from build123d import *

# Parameters (mm, degrees)
F1_DEPTH = 25.4


with BuildPart() as f1:
    # F0 (on Front) → F1 (new body)
    with BuildSketch(Plane.XZ):
        with BuildLine():
            Line((-18.234044, -41.093612), (-33.907204, -68.240322))
            ThreePointArc((-33.907204, -68.240322), (-17.414469, -74.183396), (0, -76.2))
            Line((0, -76.2), (0, -44.45))
            ThreePointArc((0, -44.45), (-9.187875, -43.490061), (-17.97891, -40.651707))
            ThreePointArc((-17.97891, -40.651707), (-18.100554, -40.876079), (-18.234044, -41.093612))
        make_face()
        with BuildLine():
            Line((0, -44.45), (0, -76.2))
            ThreePointArc((0, -76.2), (17.414469, -74.183396), (33.907204, -68.240322))
            Line((33.907204, -68.240322), (18.234044, -41.093612))
            ThreePointArc((18.234044, -41.093612), (18.100554, -40.876079), (17.97891, -40.651707))
            ThreePointArc((17.97891, -40.651707), (9.187875, -43.490061), (0, -44.45))
        make_face()
        with BuildLine():
            Line((-17.97891, -40.651707), (-18.234044, -41.093612))
            ThreePointArc((-18.234044, -41.093612), (-18.100554, -40.876079), (-17.97891, -40.651707))
        make_face()
        with BuildLine():
            Line((0, -20.6375), (0, -44.45))
            ThreePointArc((0, -44.45), (9.187875, -43.490061), (17.97891, -40.651707))
            ThreePointArc((17.97891, -40.651707), (17.659459, -37.139382), (19.84375, -34.370383))
            Line((19.84375, -34.370383), (10.31875, -17.872599))
            ThreePointArc((10.31875, -17.872599), (5.341378, -19.934294), (0, -20.6375))
        make_face()
        with BuildLine():
            ThreePointArc((-17.97891, -40.651707), (-9.187875, -43.490061), (0, -44.45))
            Line((0, -44.45), (0, -20.6375))
            ThreePointArc((0, -20.6375), (-5.341378, -19.934294), (-10.31875, -17.872599))
            Line((-10.31875, -17.872599), (-19.84375, -34.370383))
            ThreePointArc((-19.84375, -34.370383), (-17.659459, -37.139382), (-17.97891, -40.651707))
        make_face()
        with BuildLine():
            ThreePointArc((17.97891, -40.651707), (18.100554, -40.876079), (18.234044, -41.093612))
            Line((18.234044, -41.093612), (17.97891, -40.651707))
        make_face()
        with BuildLine():
            ThreePointArc((-26.215956, -35.896046), (-23.333919, -33.863231), (-19.84375, -34.370383))
            Line((-19.84375, -34.370383), (-10.31875, -17.872599))
            ThreePointArc((-10.31875, -17.872599), (-14.592916, -14.592916), (-17.872599, -10.31875))
            Line((-17.872599, -10.31875), (-38.494829, -22.225))
            ThreePointArc((-38.494829, -22.225), (-33.06956, -29.701964), (-26.215956, -35.896046))
        make_face()
        with BuildLine():
            Line((10.31875, -17.872599), (19.84375, -34.370383))
            ThreePointArc((19.84375, -34.370383), (23.333919, -33.863231), (26.215956, -35.896046))
            ThreePointArc((26.215956, -35.896046), (33.06956, -29.701964), (38.494829, -22.225))
            Line((38.494829, -22.225), (17.872599, -10.31875))
            ThreePointArc((17.872599, -10.31875), (14.592916, -14.592916), (10.31875, -17.872599))
        make_face()
        with BuildLine():
            Line((-26.47109, -36.337951), (-26.215956, -35.896046))
            ThreePointArc((-26.215956, -35.896046), (-26.349446, -36.113579), (-26.47109, -36.337951))
        make_face()
        with BuildLine():
            ThreePointArc((-26.47109, -36.337951), (-26.349446, -36.113579), (-26.215956, -35.896046))
            ThreePointArc((-26.215956, -35.896046), (-33.06956, -29.701964), (-38.494829, -22.225))
            Line((-38.494829, -22.225), (-65.991136, -38.1))
            ThreePointArc((-65.991136, -38.1), (-55.537471, -52.173071), (-42.14425, -63.484661))
            Line((-42.14425, -63.484661), (-26.47109, -36.337951))
        make_face()
        with BuildLine():
            ThreePointArc((38.494829, -22.225), (33.06956, -29.701964), (26.215956, -35.896046))
            ThreePointArc((26.215956, -35.896046), (26.349446, -36.113579), (26.47109, -36.337951))
            Line((26.47109, -36.337951), (42.14425, -63.484661))
            ThreePointArc((42.14425, -63.484661), (55.537471, -52.173071), (65.991136, -38.1))
            Line((65.991136, -38.1), (38.494829, -22.225))
        make_face()
        with BuildLine():
            ThreePointArc((26.47109, -36.337951), (26.349446, -36.113579), (26.215956, -35.896046))
            Line((26.215956, -35.896046), (26.47109, -36.337951))
        make_face()
        with BuildLine():
            Line((-38.494829, -22.225), (-17.872599, -10.31875))
            ThreePointArc((-17.872599, -10.31875), (-19.934294, -5.341378), (-20.6375, 0))
            Line((-20.6375, 0), (-39.6875, 0))
            ThreePointArc((-39.6875, 0), (-40.993377, -3.276151), (-44.194866, -4.755661))
            ThreePointArc((-44.194866, -4.755661), (-42.257436, -13.788097), (-38.494829, -22.225))
        make_face()
        with BuildLine():
            ThreePointArc((20.6375, 0), (19.934294, -5.341378), (17.872599, -10.31875))
            Line((17.872599, -10.31875), (38.494829, -22.225))
            ThreePointArc((38.494829, -22.225), (42.257436, -13.788097), (44.194866, -4.755661))
            ThreePointArc((44.194866, -4.755661), (40.993377, -3.276151), (39.6875, 0))
            Line((39.6875, 0), (20.6375, 0))
        make_face()
        with BuildLine():
            Line((0, 44.45), (0, 20.6375))
            ThreePointArc((0, 20.6375), (5.341378, 19.934294), (10.31875, 17.872599))
            Line((10.31875, 17.872599), (19.84375, 34.370383))
            ThreePointArc((19.84375, 34.370383), (17.659459, 37.139382), (17.97891, 40.651707))
            ThreePointArc((17.97891, 40.651707), (9.187875, 43.490061), (0, 44.45))
        make_face()
        with BuildLine():
            ThreePointArc((-10.31875, 17.872599), (-5.341378, 19.934294), (0, 20.6375))
            Line((0, 20.6375), (0, 44.45))
            ThreePointArc((0, 44.45), (-9.187875, 43.490061), (-17.97891, 40.651707))
            ThreePointArc((-17.97891, 40.651707), (-17.659459, 37.139382), (-19.84375, 34.370383))
            Line((-19.84375, 34.370383), (-10.31875, 17.872599))
        make_face()
        with BuildLine():
            ThreePointArc((17.872599, 10.31875), (19.934294, 5.341378), (20.6375, 0))
            Line((20.6375, 0), (39.6875, 0))
            ThreePointArc((39.6875, 0), (40.993377, 3.276151), (44.194866, 4.755661))
            ThreePointArc((44.194866, 4.755661), (42.257436, 13.788097), (38.494829, 22.225))
            Line((38.494829, 22.225), (17.872599, 10.31875))
        make_face()
        with BuildLine():
            Line((-39.6875, 0), (-20.6375, 0))
            ThreePointArc((-20.6375, 0), (-19.934294, 5.341378), (-17.872599, 10.31875))
            Line((-17.872599, 10.31875), (-38.494829, 22.225))
            ThreePointArc((-38.494829, 22.225), (-42.257436, 13.788097), (-44.194866, 4.755661))
            ThreePointArc((-44.194866, 4.755661), (-40.993377, 3.276151), (-39.6875, 0))
        make_face()
        with BuildLine():
            ThreePointArc((-17.872599, 10.31875), (-14.592916, 14.592916), (-10.31875, 17.872599))
            Line((-10.31875, 17.872599), (-19.84375, 34.370383))
            ThreePointArc((-19.84375, 34.370383), (-23.333919, 33.863231), (-26.215956, 35.896046))
            ThreePointArc((-26.215956, 35.896046), (-33.06956, 29.701964), (-38.494829, 22.225))
            Line((-38.494829, 22.225), (-17.872599, 10.31875))
        make_face()
        with BuildLine():
            Line((19.84375, 34.370383), (10.31875, 17.872599))
            ThreePointArc((10.31875, 17.872599), (14.592916, 14.592916), (17.872599, 10.31875))
            Line((17.872599, 10.31875), (38.494829, 22.225))
            ThreePointArc((38.494829, 22.225), (33.06956, 29.701964), (26.215956, 35.896046))
            ThreePointArc((26.215956, 35.896046), (23.333919, 33.863231), (19.84375, 34.370383))
        make_face()
        with BuildLine():
            Line((-65.991136, -38.1), (-38.494829, -22.225))
            ThreePointArc((-38.494829, -22.225), (-42.257436, -13.788097), (-44.194866, -4.755661))
            ThreePointArc((-44.194866, -4.755661), (-44.45, -4.7625), (-44.705134, -4.755661))
            Line((-44.705134, -4.755661), (-76.051454, -4.755661))
            ThreePointArc((-76.051454, -4.755661), (-72.95194, -22.010325), (-65.991136, -38.1))
        make_face()
        with BuildLine():
            ThreePointArc((44.194866, -4.755661), (42.257436, -13.788097), (38.494829, -22.225))
            Line((38.494829, -22.225), (65.991136, -38.1))
            ThreePointArc((65.991136, -38.1), (72.95194, -22.010325), (76.051454, -4.755661))
            Line((76.051454, -4.755661), (44.705134, -4.755661))
            ThreePointArc((44.705134, -4.755661), (44.45, -4.7625), (44.194866, -4.755661))
        make_face()
        with BuildLine():
            ThreePointArc((-17.97891, 40.651707), (-9.187875, 43.490061), (0, 44.45))
            Line((0, 44.45), (0, 76.2))
            ThreePointArc((0, 76.2), (-17.414469, 74.183396), (-33.907204, 68.240322))
            Line((-33.907204, 68.240322), (-18.234044, 41.093612))
            ThreePointArc((-18.234044, 41.093612), (-18.100554, 40.876079), (-17.97891, 40.651707))
        make_face()
        with BuildLine():
            Line((0, 76.2), (0, 44.45))
            ThreePointArc((0, 44.45), (9.187875, 43.490061), (17.97891, 40.651707))
            ThreePointArc((17.97891, 40.651707), (18.100554, 40.876079), (18.234044, 41.093612))
            Line((18.234044, 41.093612), (33.907204, 68.240322))
            ThreePointArc((33.907204, 68.240322), (17.414469, 74.183396), (0, 76.2))
        make_face()
        with BuildLine():
            ThreePointArc((-44.194866, 4.755661), (-42.257436, 13.788097), (-38.494829, 22.225))
            Line((-38.494829, 22.225), (-65.991136, 38.1))
            ThreePointArc((-65.991136, 38.1), (-72.95194, 22.010325), (-76.051454, 4.755661))
            Line((-76.051454, 4.755661), (-44.705134, 4.755661))
            ThreePointArc((-44.705134, 4.755661), (-44.45, 4.7625), (-44.194866, 4.755661))
        make_face()
        with BuildLine():
            Line((-65.991136, 38.1), (-38.494829, 22.225))
            ThreePointArc((-38.494829, 22.225), (-33.06956, 29.701964), (-26.215956, 35.896046))
            ThreePointArc((-26.215956, 35.896046), (-26.349446, 36.113579), (-26.47109, 36.337951))
            Line((-26.47109, 36.337951), (-42.14425, 63.484661))
            ThreePointArc((-42.14425, 63.484661), (-55.537471, 52.173071), (-65.991136, 38.1))
        make_face()
        with BuildLine():
            ThreePointArc((26.215956, 35.896046), (33.06956, 29.701964), (38.494829, 22.225))
            Line((38.494829, 22.225), (65.991136, 38.1))
            ThreePointArc((65.991136, 38.1), (55.537471, 52.173071), (42.14425, 63.484661))
            Line((42.14425, 63.484661), (26.47109, 36.337951))
            ThreePointArc((26.47109, 36.337951), (26.349446, 36.113579), (26.215956, 35.896046))
        make_face()
        with BuildLine():
            Line((65.991136, 38.1), (38.494829, 22.225))
            ThreePointArc((38.494829, 22.225), (42.257436, 13.788097), (44.194866, 4.755661))
            ThreePointArc((44.194866, 4.755661), (44.45, 4.7625), (44.705134, 4.755661))
            Line((44.705134, 4.755661), (76.051454, 4.755661))
            ThreePointArc((76.051454, 4.755661), (72.95194, 22.010325), (65.991136, 38.1))
        make_face()
        with BuildLine():
            ThreePointArc((-44.705134, -4.755661), (-44.45, -4.7625), (-44.194866, -4.755661))
            Line((-44.194866, -4.755661), (-44.705134, -4.755661))
        make_face()
        with BuildLine():
            Line((44.705134, -4.755661), (44.194866, -4.755661))
            ThreePointArc((44.194866, -4.755661), (44.45, -4.7625), (44.705134, -4.755661))
        make_face()
        with BuildLine():
            ThreePointArc((18.234044, 41.093612), (18.100554, 40.876079), (17.97891, 40.651707))
            Line((17.97891, 40.651707), (18.234044, 41.093612))
        make_face()
        with BuildLine():
            Line((-18.234044, 41.093612), (-17.97891, 40.651707))
            ThreePointArc((-17.97891, 40.651707), (-18.100554, 40.876079), (-18.234044, 41.093612))
        make_face()
        with BuildLine():
            ThreePointArc((44.705134, 4.755661), (44.45, 4.7625), (44.194866, 4.755661))
            Line((44.194866, 4.755661), (44.705134, 4.755661))
        make_face()
        with BuildLine():
            Line((-44.705134, 4.755661), (-44.194866, 4.755661))
            ThreePointArc((-44.194866, 4.755661), (-44.45, 4.7625), (-44.705134, 4.755661))
        make_face()
        with BuildLine():
            ThreePointArc((-26.47109, 36.337951), (-26.349446, 36.113579), (-26.215956, 35.896046))
            Line((-26.215956, 35.896046), (-26.47109, 36.337951))
        make_face()
        with BuildLine():
            Line((26.47109, 36.337951), (26.215956, 35.896046))
            ThreePointArc((26.215956, 35.896046), (26.349446, 36.113579), (26.47109, 36.337951))
        make_face()
    extrude(amount=F1_DEPTH)


solid = f1.part
Could you check a few things on this model? Use its own coordinates, in mm. A direction names the side the tool comes from. Coordinates: 2 decimals unless noted, no trailing zeros. Write each loop counter-clockwise with the first axis right and the second up, starting at its lowest first coordinate (ties: lowest second). Pieces come first, ordered by that corner, then holes. Notation, with made-up numbers: (43, -3.75) - (69, -3.75) arc R23 cw to (69, 22.25) - close; hole circle Ø8 at (-37.75, 55). An arc over 180 degrees is marked (long way). Put each result on its own line as item: value. Start each with the question number.
Q1. I want a section at B-B on z = -53. Write out the boundary of the cut face in (x, y), plus the area to 3 significant figures.
Q2. I want a section at D-D on z = 60.5. Write out the boundary of the cut face in (x, y).
Q3. Please list where these lines run through material, in increasing order: L1, parallel to X at y = -17.5, z = 49; L2, parallel to X at y = -6.5, z = 46.5; L3, parallel to X at y = -14.25, z = 0.5.
Q4. I want a section at A-A on x = 47. Write out the boundary of the cut face in (y, z), plus the area to 3 significant figures.
Q5. Which directions (+Z, -Z, +X, -X, +Y, -Y) give clear straight access to the entire face, cutting with the end or side of a thin tool? Please do faces 1 (the flat face through (-60, -13, -4.756)), 2 (the flat face through (16, 0, -16)), 3 (the flat face through (60, -13, -4.756)).
Q6. I want a section at C-C on z = 12.5. Write out the boundary of the cut face in (x, y), plus the area to 3 significant figures.
Q7. I'm going to push flat-ended pins straight in: P1, Ø1, axis at x = -24, y = -10.5, coming from the +Z side; P2, Ø12.5, axis at x = 59.5, y = -14.5, coming from the +Z side; P3, Ø10, axis at y = -5.5, z = -11, coming from the +X side. Where does each tip first touch, or does it pass through?
Q8. Thinking about a two-plate mould opening in Z: for faces 4 (the flat face through (16, -25.4, -16)), 5 (the cylindrical face through (55.37, -12.52, -52.35)), 6 (the flat face through (60, -13, 4.756)), 7 (the flat face through (-60, -13, 4.756)), which applies, pulls with the +Z half, pulls with the -Z half, needs draft (parallel to the pull), parting line crosses it, or undercut?
Checks:
1. outline: (-54.75, -25.4) - (-36.09, -25.4) - (-36.09, 0) - (-54.75, 0) - close; (-25.11, -25.4) - (25.11, -25.4) - (25.11, 0) - (-25.11, 0) - close; (36.09, -25.4) - (54.75, -25.4) - (54.75, 0) - (36.09, 0) - close
1. area: 2,220 mm²
2. outline: (-46.33, -25.4) - (-40.42, -25.4) - (-40.42, 0) - (-46.33, 0) - close; (-29.44, -25.4) - (29.44, -25.4) - (29.44, 0) - (-29.44, 0) - close; (40.42, -25.4) - (46.33, -25.4) - (46.33, 0) - (40.42, 0) - close
3. L1: -58.36 to -33.78, -22.8 to 22.8, 33.78 to 58.36
3. L2: -60.37 to -32.34, -21.36 to 21.36, 32.34 to 60.37
3. L3: -39.71 to -20.63, 20.63 to 39.71
4. outline: (-25.4, -59.98) - (0, -59.98) - (0, -4.76) - (-25.4, -4.76) - close; (-25.4, 4.76) - (0, 4.76) - (0, 59.98) - (-25.4, 59.98) - close
4. area: 2,810 mm²
5. face 1: -X, +Y, -Y
5. face 2: +Z, -Z, +X, -X, +Y
5. face 3: +X, +Y, -Y
6. outline: (-75.17, -25.4) - (-16.42, -25.4) - (-16.42, 0) - (-75.17, 0) - close; (16.42, -25.4) - (75.17, -25.4) - (75.17, 0) - (16.42, 0) - close
6. area: 2,980 mm²
7. P1: z = 72.49
7. P2: z = 54.51
7. P3: x = 75.96
8. face 4: needs draft
8. face 5: pulls with the -Z half
8. face 6: undercut
8. face 7: undercut
